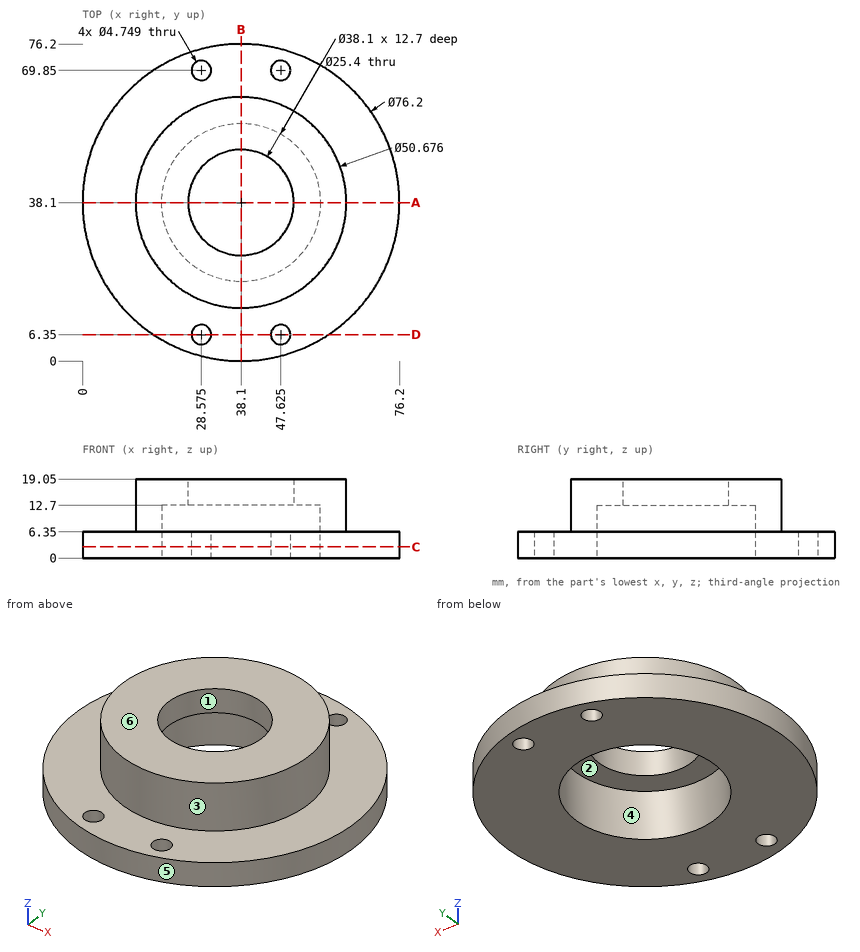
Geometry: see drawing. Coordinates: mm, zero at the bounding-box minimum. A direction names the side the tool comes from. Give positions to 0.01 mm unless a question says otherwise; leave off trailing zeros. Write each loop counter-clockwise with the first axis right and the second up, starting at its lowest first coordinate (ties: lowest second). Pieces come first, ordered by that corner, then holes. Notation, with made-up numbers: M -17.5,-22.75 L 36.5,-22.75 A13 cw 36.5,-13.75 Z; hole C 49.5,-36.75 d9. An arc over 180 degrees is marked long. Answer in a Markdown table with one row per item. Add a question column.
(1) Reachability of the marked faces 1, 2 and 3 from +Z, -Z, +X, -X, +Y, -Y: full face, straight path, thin tool, end or side. Return the list, or none.
(2) Section C-C on z = 2.75. State how many separate pieces and enclosed holes the cut face has, and give its area (3 significant figures).
(3) Section D-D on y = 6.35. Return loops of the section in (x, z), and give its area (3 significant figures).
(4) First-contact query: pin 1 (5 mm diameter, centred on x = 34.5, y = 63, fed in from -Z); pin 2 (1 mm diameter, centred on y = 37, z = 5.5, fed in from -X) (1 decimal); pin 3 (4 mm diameter, centred on x = 28.575, y = 6.35, fed in from -Z); pin 4 (6 mm diameter, centred on x = 47.625, y = 6.35, fed in from +Z). Flat tips, straight axial feed; report the tip coordinate or a pass-through.
(5) Ray query, line 1 (X direction, y = 71.5, z = 5); line 2 (X direction, y = 5, z = 4.25); line 3 (Z direction, x = 56.5, y = 64). Return the intervals inside material, ascending.
(6) Mould query, pull axis Y, two halves, no side actions, for the marked faces 4, 5 and 6. Classes: +Y half, -Y half, draft (parallel to the pull), parting line (faces both ways), or undercut.
(7) Section A-A on y = 38.1. Return loops of the section in (x, z).
Result set:
| question | item | result |
|---|---|---|
| 1 | face 1 | +Z, -Z |
| 1 | face 2 | -Z |
| 1 | face 3 | +Z |
| 2 | separate pieces | 1 |
| 2 | enclosed holes | 5 |
| 2 | area | 3,350 mm^2 |
| 3 | outline | M 17.04,0 L 26.2,0 L 26.2,6.35 L 17.04,6.35 Z; M 30.95,0 L 45.25,0 L 45.25,6.35 L 30.95,6.35 Z; M 50,0 L 59.16,0 L 59.16,6.35 L 50,6.35 Z |
| 3 | area | 207 mm^2 |
| 4 | pin 1 | stops at z = 0 |
| 4 | pin 2 | stops at x = 0 |
| 4 | pin 3 | passes through |
| 4 | pin 4 | stops at z = 6.35 |
| 5 | line 1 | x = 19.77 to 26.87, 30.28 to 45.92, 49.33 to 56.43 |
| 5 | line 2 | x = 19.23 to 26.62, 30.53 to 45.67, 49.58 to 56.97 |
| 5 | line 3 | z = 0 to 6.35 |
| 6 | face 4 | undercut |
| 6 | face 5 | parting line |
| 6 | face 6 | draft |
| 7 | outline | M 0,0 L 19.05,0 L 19.05,12.7 L 25.4,12.7 L 25.4,19.05 L 12.76,19.05 L 12.76,6.35 L 0,6.35 Z; M 50.8,12.7 L 57.15,12.7 L 57.15,0 L 76.2,0 L 76.2,6.35 L 63.44,6.35 L 63.44,19.05 L 50.8,19.05 Z |
